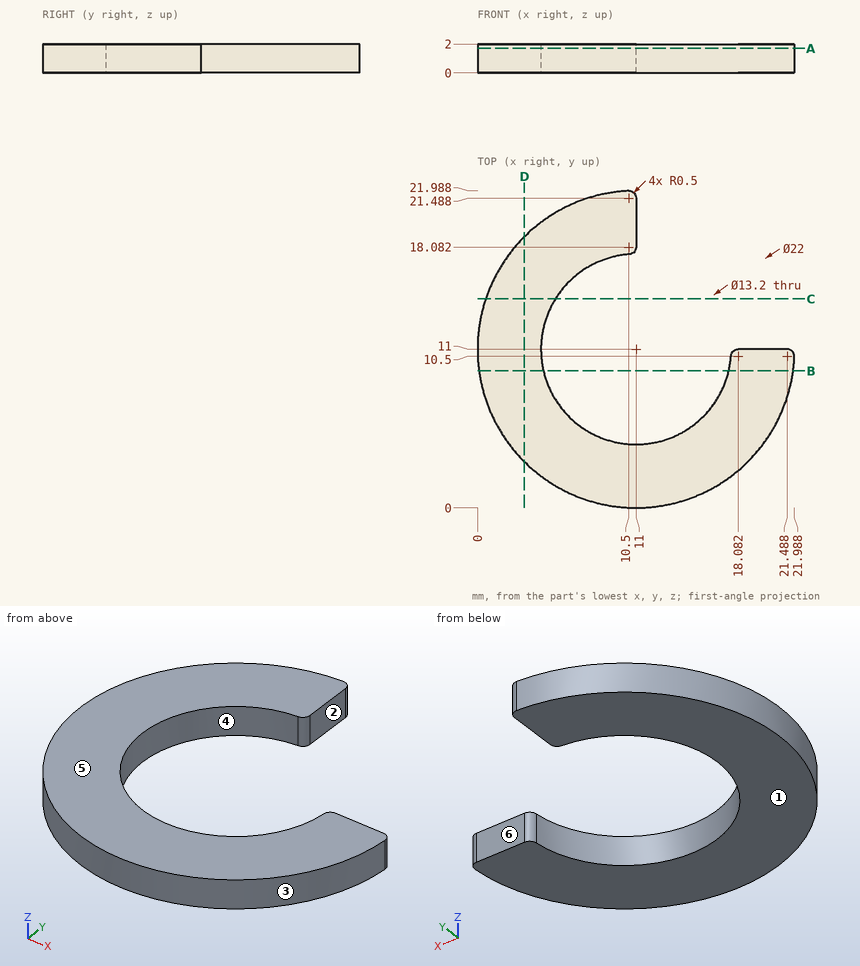
The drawing under review shows one solid part. Ordinate dimensions are in mm from its lowest x, y, z. A direction names the side the tool comes from. Coordinates: 2 decimals unless noted, no trailing zeros. Order: outer loops, then holes, each group sorted by start corner. A loop starts at its lowest first (then second) coordinate and runs counter-clockwise, first axis right, second up. Notation, with made-up numbers: (-16, 4.5) -> (36, 4.5) arc R26 ccw to (36, 35.5) -> close; hole circle Ø8 at (67.5, 55.25). An arc over 180 degrees is marked (long way). Use CSV: the item, a comma, the result in double quotes. Start each with the question number.
Item 1: Wall thickness on probe 1 along X at (y, z) = (5, 0.45); probe 2 along Y at (x, z) = (6, 0.65); probe 3 along X at (y, z) = (8, 0.5): over which ranges is each line inside the solid? List them lowest first.
Item 2: We need section D-D, the plane x = 3.25. Give the boundary of the cut face in (y, z).
Item 3: We need section C-C, the plane y = 14.5. Give the boundary of the cut face in (x, z) (1 decimal).
Item 4: For the marked faces 1 and 2, list the 3-axis set-ups (+Z, -Z, +X, -X, +Y, -Y) from which the entire face can be reached by the end or side of a thin tool; tool diameter is ignored.
Item 5: We need section A-A, the plane z = 1.7. Give the boundary of the cut face in (x, y) (1 decimal).
Item 6: Draft analysis for pull direction Y (two halves, no side actions). For the marked faces 3, 4, 5 and 6, state which applies: pulls with the +Y half, pulls with the -Y half, needs draft (parallel to the pull), parting line crosses it, or undercut.
Item 7: Insertion check: pin 1 (0.6 mm diameter, centred on x = 20, z = 0.5, fed in from +Y); pin 2 (12 mm diameter, centred on x = 11, y = 11, fed in from -Z). Each pin has a flat end and moves straight along its axis. Give the tip position at first contact, or say it passes through.
Item 8: We need section B-B, the plane y = 9.5. Give the boundary of the cut face in (x, z), then the cut area to 3 significant figures.
Derived:
1,probe 1,"x = 1.78 to 8.25, 13.75 to 20.22"
1,probe 2,"y = 1.2 to 6.69, 15.31 to 20.8"
1,probe 3,"x = 0.42 to 5.12, 16.88 to 21.58"
2,outline,"(3.19, 0) -> (18.81, 0) -> (18.81, 2) -> (3.19, 2) -> close"
3,outline,"(0.6, 0) -> (5.4, 0) -> (5.4, 2) -> (0.6, 2) -> close"
4,face 1,"-Z, +X, -X, +Y, -Y"
4,face 2,"+Z, -Z, +X, +Y"
5,outline,"(10.5, 17.6) arc R0.5 ccw to (11, 18.1) -> (11, 21.5) arc R0.5 ccw to (10.5, 22) arc R11 ccw (long way) to (22, 10.5) arc R0.5 ccw to (21.5, 11) -> (18.1, 11) arc R0.5 ccw to (17.6, 10.5) arc R6.6 cw (long way) to start"
6,face 3,"parting line crosses it"
6,face 4,"undercut"
6,face 5,"needs draft"
6,face 6,"pulls with the +Y half"
7,pin 1,"stops at y = 11"
7,pin 2,"passes through"
8,outline,"(0.1, 0) -> (4.57, 0) -> (4.57, 2) -> (0.1, 2) -> close; (17.43, 0) -> (21.9, 0) -> (21.9, 2) -> (17.43, 2) -> close"
8,area,"17.9 mm^2"
